```python
from build123d import *

# Parameters (mm, degrees)
F0_R     = 9.525
F0_R_2   = 19.05
F1_DEPTH = 25.4
F2_DEPTH = 50.8
F0_R_3   = 12.7
F3_DEPTH = 25.4


with BuildPart() as f1:
    # F0 (on Top) → F1 (new body)
    with BuildSketch(Plane.XY):
        with BuildLine():
            Line((-19.05, 25.4), (19.05, 25.4))
            ThreePointArc((19.05, 25.4), (0, 31.75), (-19.05, 25.4))
        make_face()
        with BuildLine():
            ThreePointArc((-19.114402028, -25.3515706636), (-0.0167484131, -31.7499955825), (19.0876450268, -25.3717225929))
            Line((19.0876450268, -25.3717225929), (-19.114402028, -25.3515706636))
        make_face()
        with BuildLine():
            ThreePointArc((-54.4814434441, -25.3329142257), (-52.6499961562, -25.399996466), (-50.8184791146, -25.3348464729))
            Line((-50.8184791146, -25.3348464729), (-54.4814434441, -25.3329142257))
        make_face()
        with BuildLine():
            ThreePointArc((-19.114402028, -25.3515706636), (-31.7499744369, 0.0402896446), (-19.05, 25.4))
            Line((-19.05, 25.4), (-52.6365974257, 25.4))
            ThreePointArc((-52.6365974257, 25.4), (-78.0198204414, 0.9230326826), (-54.4814434441, -25.3329142257))
            Line((-54.4814434441, -25.3329142257), (-50.8184791146, -25.3348464729))
            Line((-50.8184791146, -25.3348464729), (-19.114402028, -25.3515706636))
        make_face()
        with Locations((-52.6365974257, 0)):
            Circle(F0_R, mode=Mode.SUBTRACT)
        with BuildLine():
            ThreePointArc((19.05, 25.4), (28.3980633142, 14.1990316571), (31.75, 0))
            ThreePointArc((31.75, 0), (28.4085834705, -14.1779718295), (19.0876450268, -25.3717225929))
            Line((19.0876450268, -25.3717225929), (72.6864750945, -25.399996466))
            ThreePointArc((72.6864750945, -25.399996466), (98.0998729414, -0.0066993655), (72.6998738249, 25.4))
            Line((72.6998738249, 25.4), (19.05, 25.4))
        make_face()
        with BuildLine():
            ThreePointArc((44.1823822002, -9.4888135551), (33.8302697715, 0.2125014193), (44.6048393131, 9.4423657283))
            Line((44.6048393131, 9.4423657283), (72.544717238, 9.5249583835))
            ThreePointArc((72.544717238, 9.5249583835), (79.2981036912, 6.7451396016), (82.0978738249, 0))
            ThreePointArc((82.0978738249, 0), (79.146859724, -6.8926289903), (72.1223705392, -9.5143403234))
            Line((72.1223705392, -9.5143403234), (44.1823822002, -9.4888135551))
        make_face(mode=Mode.SUBTRACT)
        with BuildLine():
            ThreePointArc((19.0876450268, -25.3717225929), (28.4085834705, -14.1779718295), (31.75, 0))
            ThreePointArc((31.75, 0), (28.3980633142, 14.1990316571), (19.05, 25.4))
            Line((19.05, 25.4), (-19.05, 25.4))
            ThreePointArc((-19.05, 25.4), (-31.7499744369, 0.0402896446), (-19.114402028, -25.3515706636))
            Line((-19.114402028, -25.3515706636), (19.0876450268, -25.3717225929))
        make_face()
        Circle(F0_R_2, mode=Mode.SUBTRACT)
    extrude(amount=F1_DEPTH)

    # F0 (on Top) → F2 (join)
    with BuildSketch(Plane.XY):
        with BuildLine():
            ThreePointArc((19.0876450268, -25.3717225929), (28.4085834705, -14.1779718295), (31.75, 0))
            ThreePointArc((31.75, 0), (28.3980633142, 14.1990316571), (19.05, 25.4))
            Line((19.05, 25.4), (-19.05, 25.4))
            ThreePointArc((-19.05, 25.4), (-31.7499744369, 0.0402896446), (-19.114402028, -25.3515706636))
            Line((-19.114402028, -25.3515706636), (19.0876450268, -25.3717225929))
        make_face()
        Circle(F0_R_2, mode=Mode.SUBTRACT)
        with BuildLine():
            ThreePointArc((-19.114402028, -25.3515706636), (-0.0167484131, -31.7499955825), (19.0876450268, -25.3717225929))
            Line((19.0876450268, -25.3717225929), (-19.114402028, -25.3515706636))
        make_face()
        with BuildLine():
            Line((-19.05, 25.4), (19.05, 25.4))
            ThreePointArc((19.05, 25.4), (0, 31.75), (-19.05, 25.4))
        make_face()
    extrude(amount=F2_DEPTH)

    # F0 (on Top) → F3 (join)
    with BuildSketch(Plane.XY):
        Circle(F0_R_2)
        Circle(F0_R_3, mode=Mode.SUBTRACT)
    extrude(amount=F3_DEPTH)


solid = f1.part
```
Verification items for the finished model (mm, model axes). A direction names the side the tool comes from. Coordinates: 2 decimals unless noted, no trailing zeros. Write each loop counter-clockwise with the first axis right and the second up, starting at its lowest first coordinate (ties: lowest second). Pieces come first, ordered by that corner, then holes. Notation, with made-up numbers: (18, 65) - (27, 65) arc R18 ccw to (27, 86) - close; hole circle Ø3 at (-13, 78). An arc over 180 degrees is marked (long way). Write item = value, one per line.
Q1. Material ranges on L1, parallel to Y at x = 49, z = 24; L2, parallel to Y at x = 0, z = 8; L3, parallel to X at y = 8.5, z = 10, recorded low to high. Write a range as from..to.
Answer:
L1 = -25.39..-9.49, 9.46..25.4
L2 = -31.75..-12.7, 12.7..31.75
L3 = -76.57..-56.93, -48.34..-9.44, 9.44..39.05, 76.87..96.64
Q2. Mould release check, pull along X, two halves, no side actions. Record for faces 4 (the face through (4, -12.4, 25.4)), 5 (the face through (-15.12, -11.59, 37.92)), 6 (the face through (-30.586, 8.52, 30.689)), 7 (the face through (14, -14, 50.8)): released by +X, released by -X, zero draft, split by the parting line, or undercut.
Answer:
face_4 = undercut
face_5 = undercut
face_6 = split by the parting line
face_7 = zero draft
Q3. Access from +Z, -Z, +X, -X, +Y, -Y to the whole of each face (thin tool, end or side, straight path). Record for faces 1 (the face through (9, -14, 0)), 2 (the face through (46, 25.4, 13)), 3 (the face through (-36, 25.4, 13)).
Answer:
face_1 = -Z, +X, -X, +Y, -Y
face_2 = +Z, -Z, +X, +Y
face_3 = +Z, -Z, -X, +Y
Q4. Go/stop test with flat-tipped pins: pin 1 Ø15 at (x, y) = (-45, 12) entering from +Z; pin 2 Ø12 at (x, z) = (-33, 34) entering from -Y; pin 3 Ø3 at (y, z) = (19, 13) entering from -X. Record where each tip stops, or that it passes through.
Answer:
pin_1 = 25.4
pin_2 = -16.71
pin_3 = -71.05
Q5. Cross-section at A-A (z = 6). Enter the section's corners in (x, y) (3 decimals).
Answer:
outline = (-52.637, 25.4) arc R25.4 ccw (long way) to (-50.818, -25.335) - (-19.114, -25.352) arc R31.75 ccw to (19.088, -25.372) - (72.686, -25.4) arc R25.4 ccw to (72.7, 25.4) - (19.05, 25.4) arc R31.75 ccw to (-19.05, 25.4) - close; hole circle Ø19.05 at (-52.637, 0); hole circle Ø25.4 at (0, 0); hole (44.182, -9.489) - (72.122, -9.514) arc R9.525 ccw (long way) to (72.545, 9.525) - (44.605, 9.442) arc R9.525 ccw (long way) to start
Q6. Cross-section at B-B (x = 0). Enter the section's corners in (y, z).
Answer:
outline = (-31.75, 0) - (-12.7, 0) - (-12.7, 25.4) - (-19.05, 25.4) - (-19.05, 50.8) - (-31.75, 50.8) - close; (12.7, 0) - (31.75, 0) - (31.75, 50.8) - (19.05, 50.8) - (19.05, 25.4) - (12.7, 25.4) - close
Q7. Cross-section at D-D (z = 32.5). Enter the section's corners in (x, y), plus the area to 3 significant figures.
Answer:
outline = circle Ø63.5 at (0, 0); hole circle Ø38.1 at (0, 0)
area = 2,030 mm²
Q8. Cross-section at C-C (y = 3.5). Enter the section's corners in (x, z), plus the area to 3 significant figures.
Answer:
outline = (-77.79, 0) - (-61.5, 0) - (-61.5, 25.4) - (-77.79, 25.4) - close; (-43.78, 0) - (-12.21, 0) - (-12.21, 25.4) - (-18.73, 25.4) - (-18.73, 50.8) - (-31.56, 50.8) - (-31.56, 25.4) - (-43.78, 25.4) - close; (12.21, 0) - (34.49, 0) - (34.49, 25.4) - (31.56, 25.4) - (31.56, 50.8) - (18.73, 50.8) - (18.73, 25.4) - (12.21, 25.4) - close; (81.43, 0) - (97.86, 0) - (97.86, 25.4) - (81.43, 25.4) - close
area = 2,850 mm²
